```python
from build123d import *

# Parameters (mm, degrees)
BOSS_EXTRUDE1_DEPTH                                 = 22
SKETCH3_R                                           = 35
CUT_EXTRUDE1_DEPTH                                  = 18
SKETCH4_R                                           = 14
BOSS_EXTRUDE2_DEPTH                                 = 7
FILLET1_R                                           = 4
SKETCH5_R                                           = 10
CUT_EXTRUDE2_DEPTH                                  = 30
CHAMFER1_SIZE                                       = 2
M8X1_25_TAPPED_HOLE1_D                              = 6.8
M8X1_25_TAPPED_HOLE1_DEPTH                          = 29.75
M8X1_25_TAPPED_HOLE1_TIP                            = 2.042926105
CIRPATTERN1_COUNT                                   = 6
CSK_FOR_M6_COUNTERSUNK_FLAT_HEAD_SCREW2_D           = 6
CSK_FOR_M6_COUNTERSUNK_FLAT_HEAD_SCREW2_DEPTH       = 20
CSK_FOR_M6_COUNTERSUNK_FLAT_HEAD_SCREW2_CSINK_D     = 8
CSK_FOR_M6_COUNTERSUNK_FLAT_HEAD_SCREW2_CSINK_ANGLE = 90
CSK_FOR_M6_COUNTERSUNK_FLAT_HEAD_SCREW2_TIP         = 1.802581857


with BuildPart() as part:
    # Sketch2 → Boss-Extrude1 (new body)
    with BuildSketch(Plane.XY):
        with BuildLine():
            Line((-50, -59.5), (50, -59.5))
            Line((50, -59.5), (50, -49.5))
            Line((50, -49.5), (34, -49.5))
            ThreePointArc((34, -49.5), (31.171572875, -48.328427125), (30, -45.5))
            Line((30, -45.5), (30, -38.681390875))
            ThreePointArc((30, -38.681390875), (30.35561344, -37.032619635), (31.359223301, -35.677011001))
            ThreePointArc((31.359223301, -35.677011001), (47.179198283, -5.511193099), (38.737864078, 27.488686522))
            ThreePointArc((38.737864078, 27.488686522), (38.18892773, 28.588727762), (38, 29.803523282))
            Line((38, 29.803523282), (38, 47.5))
            Line((38, 47.5), (0, 47.5))
            ThreePointArc((0, 47.5), (-44.446079819, 16.756968363), (-31.359223301, -35.677011001))
            ThreePointArc((-31.359223301, -35.677011001), (-30.35561344, -37.032619635), (-30, -38.681390875))
            Line((-30, -38.681390875), (-30, -45.5))
            ThreePointArc((-30, -45.5), (-31.171572875, -48.328427125), (-34, -49.5))
            Line((-34, -49.5), (-50, -49.5))
            Line((-50, -49.5), (-50, -59.5))
        make_face()
    extrude(amount=BOSS_EXTRUDE1_DEPTH)

    # Sketch3 → Cut-Extrude1 (cut)
    with BuildSketch(Plane.XY.offset(22)):
        Circle(SKETCH3_R)
    extrude(amount=-CUT_EXTRUDE1_DEPTH, mode=Mode.SUBTRACT)

    # Sketch4 → Boss-Extrude2 (add)
    with BuildSketch(Plane(origin=(0, 0, 0), x_dir=(-1, 0, 0), z_dir=(0, 0, -1))):
        Circle(SKETCH4_R)
    extrude(amount=BOSS_EXTRUDE2_DEPTH)

    # Fillet1
    fillet1_edges = [part.edges().sort_by_distance(p)[0] for p in [
        (14, 0, 0),
    ]]
    fillet(fillet1_edges, radius=FILLET1_R)

    # Sketch5 → Cut-Extrude2 (cut, through all)
    with BuildSketch(Plane(origin=(0, 0, -7), x_dir=(-1, 0, 0), z_dir=(0, 0, -1))):
        Circle(SKETCH5_R)
    extrude(amount=-CUT_EXTRUDE2_DEPTH, mode=Mode.SUBTRACT)

    # Chamfer1
    chamfer1_edges = [part.edges().sort_by_distance(p)[0] for p in [
        (50, -54.5, 0),
        (-50, -54.5, 0),
        (-50, -54.5, 22),
        (50, -54.5, 22),
    ]]
    chamfer(chamfer1_edges, length=CHAMFER1_SIZE)

    # M8x1.25 Tapped Hole1
    with Locations(Plane(origin=(30.22415, 47.5, 11), x_dir=(0, 0, 1), z_dir=(0, 1, 0))):
        with Locations((0, 0)):
            Hole(M8X1_25_TAPPED_HOLE1_D / 2, depth=M8X1_25_TAPPED_HOLE1_DEPTH)
            with Locations((0, 0, -(M8X1_25_TAPPED_HOLE1_DEPTH + M8X1_25_TAPPED_HOLE1_TIP / 2))):  # 118° drill point
                Cone(0, M8X1_25_TAPPED_HOLE1_D / 2, M8X1_25_TAPPED_HOLE1_TIP, mode=Mode.SUBTRACT)

    # Sketch11 → M6x1.0 Tapped Hole1 (revolve, cut)
    with BuildSketch(Plane(origin=(0, 40, 22), x_dir=(0, -1, 0), z_dir=(1, 0, 0))):
        Polygon((0, 0), (0, 16.502151548), (2.5, 15), (2.5, 0), align=None)
    m6x1_0_tapped_hole1 = revolve(axis=Axis((0, 40, 28.35), (0, 0, -1)), mode=Mode.SUBTRACT)

    # CirPattern1: M6x1.0 Tapped Hole1 ×6 about axis
    cirpattern1_axis = Axis((0, 0, 0), (0, 0, 1))
    for i in range(1, CIRPATTERN1_COUNT):
        add(m6x1_0_tapped_hole1.rotate(cirpattern1_axis, i * 360 / CIRPATTERN1_COUNT), mode=Mode.SUBTRACT)

    # CSK for M6 Countersunk Flat Head Screw2
    with Locations(Plane(origin=(0, -59.5, 0), x_dir=(-1, 0, 0), z_dir=(0, -1, 0))):
        with Locations((-42, -11), (42, -11)):
            CounterSinkHole(CSK_FOR_M6_COUNTERSUNK_FLAT_HEAD_SCREW2_D / 2, CSK_FOR_M6_COUNTERSUNK_FLAT_HEAD_SCREW2_CSINK_D / 2, depth=CSK_FOR_M6_COUNTERSUNK_FLAT_HEAD_SCREW2_DEPTH, counter_sink_angle=CSK_FOR_M6_COUNTERSUNK_FLAT_HEAD_SCREW2_CSINK_ANGLE)
            with Locations((0, 0, -(CSK_FOR_M6_COUNTERSUNK_FLAT_HEAD_SCREW2_DEPTH + CSK_FOR_M6_COUNTERSUNK_FLAT_HEAD_SCREW2_TIP / 2))):  # 118° drill point
                Cone(0, CSK_FOR_M6_COUNTERSUNK_FLAT_HEAD_SCREW2_D / 2, CSK_FOR_M6_COUNTERSUNK_FLAT_HEAD_SCREW2_TIP, mode=Mode.SUBTRACT)


solid = part.part
```
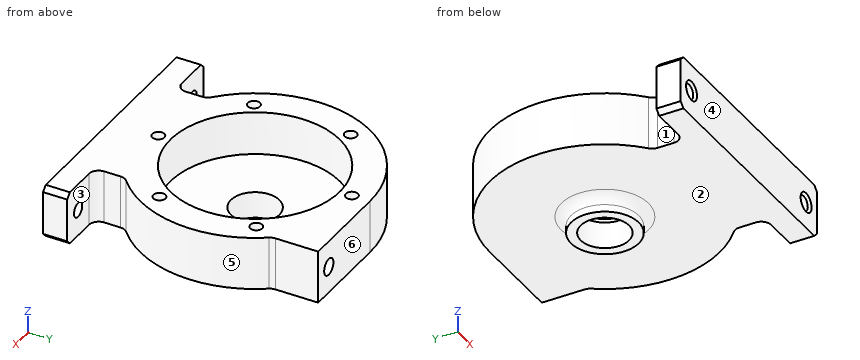
Verification items for the finished model (mm, model axes). Face numbers are marked on the shaded views. A direction names the side the tool comes from. Round coordinates to 2 decimals unless told otherwise and drop trailing zeros. Write each loop counter-clockwise with the first axis right and the second up, starting at its lowest first coordinate (ties: lowest second). Pieces come first, ordered by that corner, then holes.
1. Section check B-B on x = -42. Enter the section's corners in (y, z).
2. Scan lines: L1, parallel to X at y = -54, z = 11; L2, parallel to X at y = -20, z = 13.25; L3, parallel to Z at x = 42, y = -55. Record each from-to range of solid material in increasing order.
3. Draft check along Y on the marked faces 4, 5 and 6. Enter one of: +Y half, -Y half, draft (parallel to the pull), parting line (faces both ways), or undercut.
4. Gauge pin test, flat ends, axial feed: P1, Ø4.5, axis at x = -34.64, y = -20, coming from the -Z side; P2, Ø5, axis at x = -41, z = 11, coming from the +Y side; P3, Ø2, axis at y = -42.5, z = 9, coming from the +X side; P4, Ø12, axis at x = 0, y = 0, coming from the -Z side. Record the tip position at first contact, or that the pin passes through.
5. Section check C-C on z = 18.25. Enter the section's corners in (x, y).
6. Access from +Z, -Z, +X, -X, +Y, -Y to the whole of each face (thin tool, end or side, straight path). Record for the marked faces 1, 2 and 3.
7. Section check D-D on y = -27.5. Enter the section's corners in (x, z), plus the area to 3 significant figures.
8. Section check A-A on y = 0. Enter the section's corners in (x, z), plus the area to 3 significant figures.
Answer:
1. outline: (-59.5, 0) - (-49.5, 0) - (-49.5, 8) - (-58.5, 8) - (-59.5, 7) - close; (-59.5, 15) - (-58.5, 14) - (-49.5, 14) - (-49.5, 22) - (-59.5, 22) - close; (-22.19, 0) - (22.19, 0) - (22.19, 22) - (-22.19, 22) - close
2. L1: x = -50 to -45, -39 to 39, 45 to 50
2. L2: x = -43.08 to -37.14, -32.14 to -28.72, 28.72 to 32.14, 37.14 to 43.08
2. L3: z = 0 to 8, 14 to 22
3. face 4: -Y half
3. face 5: undercut
3. face 6: +Y half
4. P1: stops at z = 0
4. P2: stops at y = 27.82
4. P3: stops at x = 30
4. P4: passes through
5. outline: (-50, -59.5) - (50, -59.5) - (50, -49.5) - (34, -49.5) arc R4 cw to (30, -45.5) - (30, -38.68) arc R4 cw to (31.36, -35.68) arc R47.5 ccw to (38.74, 27.49) arc R4 cw to (38, 29.8) - (38, 47.5) - (0, 47.5) arc R47.5 ccw to (-31.36, -35.68) arc R4 cw to (-30, -38.68) - (-30, -45.5) arc R4 cw to (-34, -49.5) - (-50, -49.5) - close; hole circle Ø5 at (-34.64, -20); hole circle Ø5 at (-34.64, 20); hole circle Ø70 at (0, 0); hole circle Ø5 at (0, -40); hole circle Ø5 at (0, 40); hole circle Ø5 at (34.64, -20); hole circle Ø5 at (34.64, 20)
6. face 1: +Z, -Z, -X
6. face 2: -Z
6. face 3: +Z, -Z, +X
7. outline: (-38.73, 0) - (38.73, 0) - (38.73, 22) - (21.65, 22) - (21.65, 4) - (-21.65, 4) - (-21.65, 22) - (-38.73, 22) - close
7. area: 925 mm2
8. outline: (-47.5, 0) - (-18, 0) arc R4 cw to (-14, -4) - (-14, -7) - (-10, -7) - (-10, 4) - (-35, 4) - (-35, 22) - (-47.5, 22) - close; (10, -7) - (14, -7) - (14, -4) arc R4 cw to (18, 0) - (47.5, 0) - (47.5, 22) - (35, 22) - (35, 4) - (10, 4) - close
8. area: 813 mm2
